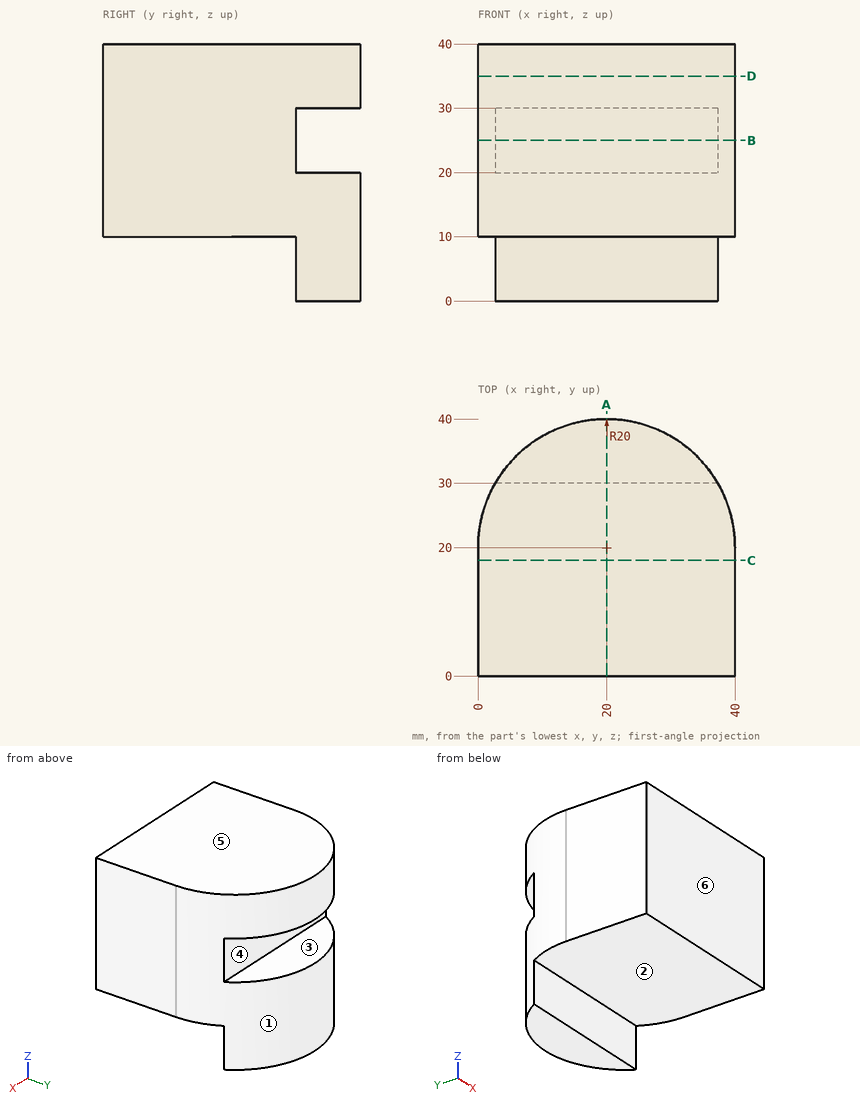
Source: three-view drawing plus pictorial views. Frame: mm from the lowest corner of the part. A direction names the side the tool comes from. Give positions to 0.01 mm unless a question says otherwise; leave off trailing zeros. Order: outer loops, then holes, each group sorted by start corner. A loop starts at its lowest first (then second) coordinate and runs counter-clockwise, first axis right, second up. Notation, with made-up numbers: (17, 64.25) -> (66, 64.25) arc R12 cw to (66, 73.25) -> close; hole circle Ø10 at (79, 56). An arc over 180 degrees is marked (long way). Write each question's results on one line, items separated by ' | '. Start each with the question number.
Item 1: Line query: line 1 (Z direction, x = 27, y = 37.5); line 2 (Z direction, x = 20, y = 25); line 3 (Y direction, x = 30, z = 9.5). Output: solid intervals per line, ascending.
Item 2: Set-up query: the marked faces 1, 2 and 3. Return all of +Z, -Z, +X, -X, +Y, -Y with unobstructed straight access to the full face (end or side cutting, diameter ignored); none if empty.
Item 3: Cut plane A-A on x = 20. Return the cut outline in (y, z).
Item 4: Cut plane D-D on z = 35. Return the cut outline in (x, y).
Item 5: Mould query, pull axis Z, two halves, no side actions, for the marked faces 4, 5 and 6. Classes: pulls with the +Z half, pulls with the -Z half, needs draft (parallel to the pull), parting line crosses it, or undercut.
Item 6: Cut plane B-B on z = 25. Return the cut outline in (x, y), then the cut area to 3 significant figures.
Item 7: Contact query for flat-ended pins moving along their axis: P1, Ø5, axis at x = 27, z = 27, coming from the +Y side; P2, Ø3, axis at x = 12, z = 3, coming from the -Y side; P3, Ø3, axis at x = 25.5, z = 12.5, coming from the +Y side. Output: stop coordinate, or through.
Item 8: Cut plane C-C on y = 18. Return the cut outline in (x, z).
Established:
1) line 1: 0 to 20, 30 to 40 | line 2: 10 to 40 | line 3: 30 to 37.32
2) face 1: +Z, -Z, +Y | face 2: -Z, +X, -X, -Y | face 3: +X, -X, +Y
3) outline: (0, 10) -> (30, 10) -> (30, 0) -> (40, 0) -> (40, 20) -> (30, 20) -> (30, 30) -> (40, 30) -> (40, 40) -> (0, 40) -> close
4) outline: (0, 0) -> (40, 0) -> (40, 20) arc R20 ccw to (0, 20) -> close
5) face 4: undercut | face 5: pulls with the +Z half | face 6: needs draft
6) outline: (0, 0) -> (40, 0) -> (40, 20) arc R20 ccw to (37.32, 30) -> (2.68, 30) arc R20 ccw to (0, 20) -> close | area: 1,180 mm^2
7) P1: y = 30 | P2: y = 30 | P3: y = 39.6
8) outline: (0, 10) -> (40, 10) -> (40, 40) -> (0, 40) -> close
